```python
from build123d import *

# Parameters (mm, degrees)
SKETCH_R  = 2.5
PAD_DEPTH = 2


with BuildPart() as part:
    # Sketch → Pad (new body)
    with BuildSketch(Plane.XY):
        Polygon((-171.233897, 259.917405), (155.766103, 259.917405), (215.766103, 199.917405), (215.766103, -210.082595), (155.766103, -270.082595), (-171.233897, -270.082595), (-231.233897, -210.082595), (-231.233897, 199.917405), align=None)
        with Locations((-220.426407, 191.551941)):
            Circle(SKETCH_R, mode=Mode.SUBTRACT)
        with Locations((-156.405304, 253.931473)):
            Circle(SKETCH_R, mode=Mode.SUBTRACT)
        with Locations((145.682602, 255.015823)):
            Circle(SKETCH_R, mode=Mode.SUBTRACT)
        with Locations((-219.194855, -200.60849)):
            Circle(SKETCH_R, mode=Mode.SUBTRACT)
        with Locations((-153.602219, -263.909698)):
            Circle(SKETCH_R, mode=Mode.SUBTRACT)
        with Locations((141.603378, -261.699738)):
            Circle(SKETCH_R, mode=Mode.SUBTRACT)
        with Locations((204.925644, -200.476547)):
            Circle(SKETCH_R, mode=Mode.SUBTRACT)
        with Locations((207.374741, 191.907639)):
            Circle(SKETCH_R, mode=Mode.SUBTRACT)
    extrude(amount=PAD_DEPTH)


solid = part.part
```
Work out the finished part from the listing and answer in its coordinate system (mm). Coordinates: 2 decimals unless noted, no trailing zeros. Write each loop counter-clockwise with the first axis right and the second up, starting at its lowest first coordinate (ties: lowest second). Pieces come first, ordered by that corner, then holes. Notation, with made-up numbers: (-39, 15) - (9, 15) arc R35 cw to (9, 47) - close; hole circle Ø6 at (80.25, 30). An arc over 180 degrees is marked (long way). Answer as a JSON object with one key per item and string values.
Q1. Consider L1, parallel to Y at x = 144.5, z = 1.55; L2, parallel to Y at x = -157.5, z = 1; L3, parallel to Y at x = 163.5, z = 0.3. Determine where each line is inside the solid, lowest interval first. Write a range as from..to.
Results list:
{"L1": "y = -270.08..252.81, 257.22..259.92", "L2": "y = -270.08..251.68, 256.18..259.92", "L3": "y = -262.35..252.18"}
Q2. Find section B-B (x = 167). Write down the section's boundary in (y, z), plus the area to 3 significant figures.
Results list:
{"outline": "(-258.85, 0) - (248.68, 0) - (248.68, 2) - (-258.85, 2) - close", "area": "1,020 mm^2"}
Q3. For a pull along Z with two mould halves and no side action, classify faces 1 (the flat face through (-5, -1, 0)), 2 (the flat face through (-5, -1, 2)), 3 (the flat face through (-201.65, 229.5, 0.99)) as pulls with the +Z half, pulls with the -Z half, needs draft (parallel to the pull), parting line crosses it, or undercut.
Results list:
{"face 1": "pulls with the -Z half", "face 2": "pulls with the +Z half", "face 3": "needs draft"}
Q4. Find section A-A (z = 0.85). State how many separate pieces and enclosed holes the cut face has, plus the area to 3 significant figures.
Results list:
{"separate pieces": "1", "enclosed holes": "8", "area": "230,000 mm^2"}
Q5. Given pin 1 Ø6.5 at (x, y) = (145.68, 255.02) entering from -Z; pin 2 Ø4 at (x, y) = (-153.6, -263.91) entering from +Z, each flat-ended and moving along its own axis, determine where each tip first touches the part or whether it passes through.
Results list:
{"pin 1": "stops at z = 0", "pin 2": "passes through"}
